```python
from build123d import *

# Parameters (mm, degrees)
SKETCH_1_W             = 42
SKETCH_1_H             = 42
EXTRUDE_1_DEPTH        = 34
HOLE_WIZARD_M3_1_D     = 2.5
HOLE_WIZARD_M3_1_DEPTH = 5
HOLE_WIZARD_M3_1_TIP   = 0.751075774
EXTRUDE_2_DEPTH        = 23
FILLET_1_R             = 5


with BuildPart() as part:
    # 草图1 → 凸台-拉伸1 (new body)
    with BuildSketch(Plane(origin=(0, 0, 0), x_dir=(1, 0, 0), z_dir=(0, 1, 0))):
        Rectangle(SKETCH_1_W, SKETCH_1_H)
    extrude(amount=EXTRUDE_1_DEPTH)

    # M3 螺纹孔1
    with Locations(Plane(origin=(0, 34, 0), x_dir=(1, 0, 0), z_dir=(0, 1, 0))):
        with Locations((-15.5, 15.5), (15.5, -15.5), (-15.5, -15.5), (15.5, 15.5)):
            Hole(HOLE_WIZARD_M3_1_D / 2, depth=HOLE_WIZARD_M3_1_DEPTH)
            with Locations((0, 0, -(HOLE_WIZARD_M3_1_DEPTH + HOLE_WIZARD_M3_1_TIP / 2))):  # 118° drill point
                Cone(0, HOLE_WIZARD_M3_1_D / 2, HOLE_WIZARD_M3_1_TIP, mode=Mode.SUBTRACT)

    # 草图5 → 凸台-拉伸2 (add)
    with BuildSketch(Plane(origin=(0, 34, 0), x_dir=(1, 0, 0), z_dir=(0, 1, 0))):
        with BuildLine():
            Line((1.984567922, 1.520358564), (-1.984567922, 1.520358564))
            ThreePointArc((-1.984567922, 1.520358564), (-0.802676832, -2.367638043), (2.5, 0))
            ThreePointArc((2.5, 0), (2.367638043, 0.802676832), (1.984567922, 1.520358564))
        make_face()
    extrude(amount=EXTRUDE_2_DEPTH)

    # 圆角1
    fillet_1_edges = [part.edges().sort_by_distance(p)[0] for p in [
        (21, 17, 21),
        (-21, 17, 21),
        (-21, 17, -21),
        (21, 17, -21),
    ]]
    fillet(fillet_1_edges, radius=FILLET_1_R)


solid = part.part
```
Input: part model. Units: mm. Frame: model coordinates. A direction names the side the tool comes from. Round coordinates to 2 decimals unless told otherwise and drop trailing zeros. Loops run counter-clockwise (first coordinate to the right, second up) from the corner with the lowest first, then second, coordinate; pieces in that order, holes last.
1) Set-up query: faces 1 (the cylindrical face through (19, 17, -20)), 2 (the cylindrical face through (-15.34, 31.46, 14.26)), 3 (the flat face through (0, 45, -1.52)). Return all of +Z, -Z, +X, -X, +Y, -Y with unobstructed straight access to the full face (end or side cutting, diameter ignored); none if empty.
Ans:
face 1: -Z, +X, +Y, -Y
face 2: +Y
face 3: -Z, +X, -X, +Y
2) Section query D-D on z = -3. Return the cut outline in (x, y), plus the area to 3 significant figures.
Ans:
outline: (-21, 0) - (21, 0) - (21, 34) - (-21, 34) - close
area: 1,430 mm2
3) Section query A-A on y = 30.5. Return the cut outline in (x, z).
Ans:
outline: (-21, -16) arc R5 ccw to (-16, -21) - (16, -21) arc R5 ccw to (21, -16) - (21, 16) arc R5 ccw to (16, 21) - (-16, 21) arc R5 ccw to (-21, 16) - close; hole circle Ø2.5 at (-15.5, -15.5); hole circle Ø2.5 at (-15.5, 15.5); hole circle Ø2.5 at (15.5, -15.5); hole circle Ø2.5 at (15.5, 15.5)
4) Section query B-B on x = 0. Return the cut outline in (y, z), plus the area to 3 significant figures.
Ans:
outline: (0, -21) - (34, -21) - (34, -1.52) - (57, -1.52) - (57, 2.5) - (34, 2.5) - (34, 21) - (0, 21) - close
area: 1,520 mm2
5) Pull-direction query (X, two-part tool) for faces 4 (the flat face through (0, 34, -5)), 5 (the cylindrical face through (15.66, 31.46, 14.26)), 6 (the flat face through (-21, 17, 0)); classes: released by +X, released by -X, zero draft, split by the parting line, or undercut.
Ans:
face 4: zero draft
face 5: undercut
face 6: released by -X
6) Material intervals for line 1 (X direction, y = 31.5, z = -15.5); line 2 (X direction, y = 31, z = 15), sorted ascending.
Ans:
line 1: x = -21 to -16.75, -14.25 to 14.25, 16.75 to 21
line 2: x = -21 to -16.65, -14.35 to 14.35, 16.65 to 21
7) Section query C-C on y = 40. Return the cut outline in (x, z), plus the area to 3 significant figures.
Ans:
outline: (-1.98, -1.52) - (1.98, -1.52) arc R2.5 ccw (long way) to start
area: 16.9 mm2
8) Pin query (flat end, axial travel): pin 1 (4 mm diameter, centred on x = 8.5, z = -1.5, fed in from +Y); pin 2 (2 mm diameter, centred on x = 15.5, z = -15.5, fed in from +Y); pin 3 (3 mm diameter, centred on x = -0.5, y = 40, fed in from -Z). Return the tip coordinate at first contact, or that it passes through.
Ans:
pin 1: stops at y = 34
pin 2: stops at y = 28.85
pin 3: stops at z = -1.52
